Geometry check sheet. Reference: the model listing, model coordinates, mm. Coordinates: 2 decimals unless noted, no trailing zeros. Write each loop counter-clockwise with the first axis right and the second up, starting at its lowest first coordinate (ties: lowest second). Pieces come first, ordered by that corner, then holes. Notation, with made-up numbers: M -0.5,87 L 3.5,87 A13 cw 3.5,109 Z; hole C -5.75,81.5 d7. An arc over 180 degrees is marked long. Answer as a JSON object with one key per item and string values. Group by question number.
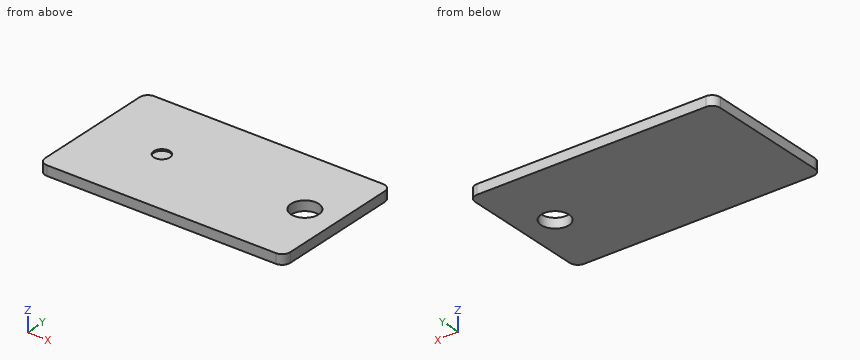
Autodesk Inventor part; units mm, degrees
ref_plane "YZ Plane" through (0, 0, 0) normal (1, 0, 0) x (0, 1, 0)
ref_plane "XZ Plane" through (0, 0, 0) normal (0, 1, 0) x (-1, 0, 0)
ref_plane "XY Plane" through (0, 0, 0) normal (0, 0, 1) x (1, 0, 0)
sketch "Sketch1" plane through (0, 0, 0) normal (0, 0, 1) x (1, 0, 0)
  line L0 (-75, -42.5) -> (75, -42.5)
  line L1 (75, -42.5) -> (75, 42.5)
  line L2 (75, 42.5) -> (-75, 42.5)
  line L3 (-75, 42.5) -> (-75, -42.5)
  line L4 (-75, -42.5) -> (75, 42.5) construction
  line L5 (75, -42.5) -> (-75, 42.5) construction
  circle A0 centre (55, -22.5) radius 8.5
  circle A1 centre (55, 22.5) radius 8.5
  line L6 (0, 0) -> (75, 0) construction
  circle A2 centre (55, 0) radius 8.5
  dimension "d0" = 150
  dimension "d1" = 85
  dimension "d23" = 17
  dimension "d25" = 20
  dimension "d26" = 20
extrude "Plate1" add sketch "Sketch1" along normal blind 6 contours L3 L2 L1 L0 | A0 | A1
sketch "Sketch5" plane through (0, 0, 6) normal (0, 0, 1) x (1, 0, 0)
  line L0 (75, -42.5) -> (-75, -42.5)
  line L1 (-75, -42.5) -> (-75, 42.5)
  line L2 (-75, 42.5) -> (75, 42.5)
  circle A0 centre (-32.5, 0) radius 42.5
  circle A1 centre (-32.5, 0) radius 5
  point P0 (0, 0)
  point P1 (50, -55)
  point P2 (-50, -55)
  point P3 (-70, -35)
  point P4 (-70, 35)
  point P5 (-50, 55)
  point P6 (50, 55)
  dimension "d27" = 10
extrude "Extrusion2" cut sketch "Sketch5" against normal blind 1 contours A1
fillet "Corner Round2" radius 5 4 edges at (-75, 42.5, 3) (-75, -42.5, 3) (75, -42.5, 3) (75, 42.5, 3)
equation "\"d26\" = d25"
equation "\"d2\" = Thickness"
equation "\"BendReliefWidth\" = Thickness"
equation "\"BendReliefDepth\" = 0.5 * Thickness"
equation "\"CornerReliefSize\" = 4 * Thickness"
equation "\"MinimumRemnant\" = 2 * Thickness"
equation "\"TransitionRadius\" = BendRadius"
equation "\"JacobiRadiusSize\" = BendRadius"
equation "\"GapSize\" = Thickness"
properties part number "PNS 1695 leg floor plate" material "Stainless Steel"
1) Go/stop test with a flat-tipped pin: pin 1 Ø6 at (x, y) = (-32.5, 0) entering from +Z. Record where the tip stops, or that it passes through.
2) Section check D-D (x = -32.5). Record the cut outline in (y, z), then the cut area to 3 significant figures.
3) Section check B-B (x = 55). Record the cut outline in (y, z), then the cut area to 3 significant figures.
4) Section check C-C (z = 2.25). Record the cut outline in (x, y).
5) Section check A-A (y = 0). Record the cut outline in (x, z).
6) Material ranges on probe 1 along Y at (x, z) = (-32.5, 5.5); probe 2 along X at (y, z) = (1, 5.25); probe 3 along X at (y, z) = (3.5, 3.15), recorded low to high. Write a range as [from, to].
Entries:
{
 "1": {"pin 1": "z = 5"},
 "2": {"outline": "M -42.5,0 L 42.5,0 L 42.5,6 L 5,6 L 5,5 L -5,5 L -5,6 L -42.5,6 Z", "area": "500 mm^2"},
 "3": {"outline": "M -42.5,0 L -8.5,0 L -8.5,6 L -42.5,6 Z; M 8.5,0 L 42.5,0 L 42.5,6 L 8.5,6 Z", "area": "408 mm^2"},
 "4": {"outline": "M -75,-37.5 A5 ccw -70,-42.5 L 70,-42.5 A5 ccw 75,-37.5 L 75,37.5 A5 ccw 70,42.5 L -70,42.5 A5 ccw -75,37.5 Z; hole C 55,0 d17"},
 "5": {"outline": "M -75,0 L 46.5,0 L 46.5,6 L -27.5,6 L -27.5,5 L -37.5,5 L -37.5,6 L -75,6 Z; M 63.5,0 L 75,0 L 75,6 L 63.5,6 Z"},
 "6": {"probe 1": "[-42.5, -5], [5, 42.5]", "probe 2": "[-75, -37.4], [-27.6, 46.56], [63.44, 75]", "probe 3": "[-75, 47.25], [62.75, 75]"}
}
